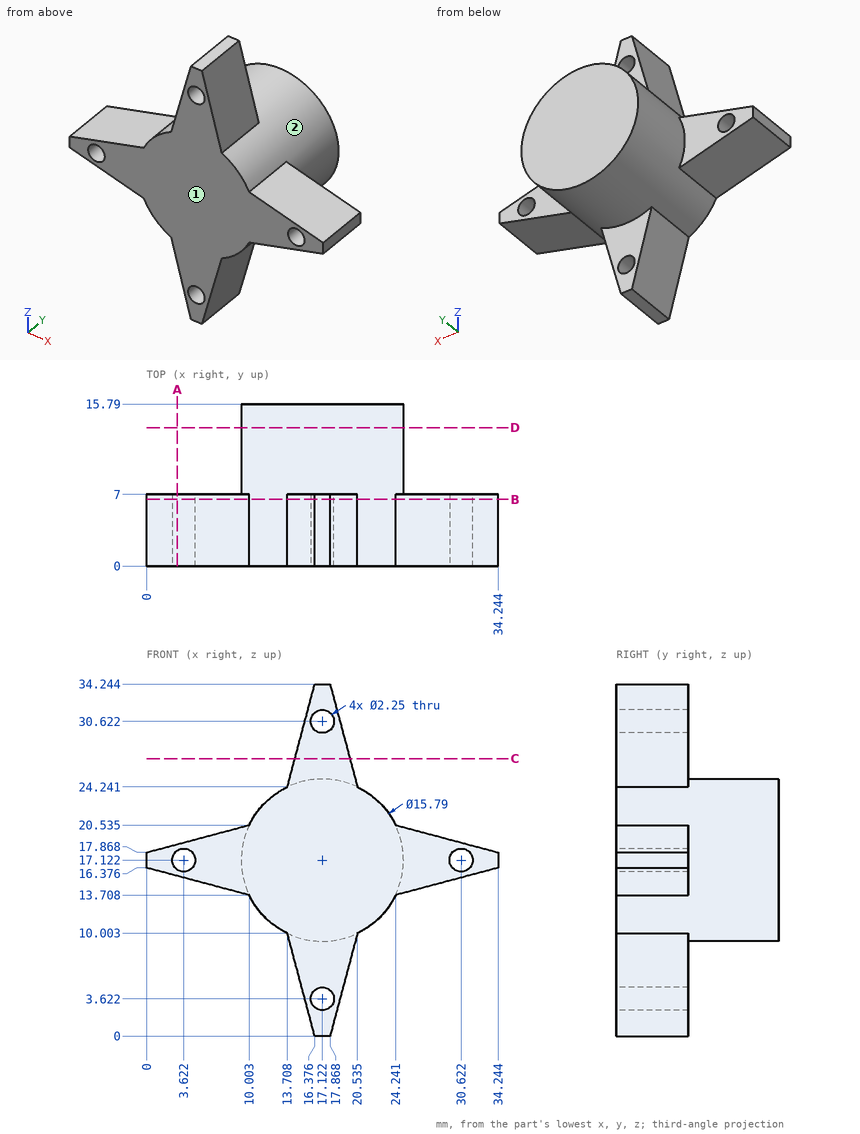
Verification items for this drawing (mm, ordinates from the low corner). A direction names the side the tool comes from. Give positions to 0.01 mm unless a question says otherwise; leave off trailing zeros. Loops run counter-clockwise (first coordinate to the right, second up) from the corner with the lowest first, then second, coordinate; pieces in that order, holes last. Notation, with made-up numbers: M 16.5,-9 L 40.5,-9 A24 ccw 40.5,27 Z; hole C 2.25,53.25 d9. An arc over 180 degrees is marked long. Return JSON: item names as keys, results as strings. Group by question number.
1. Thickness scan on L1, parallel to Y at x = 16, z = 8.5; L2, parallel to Z at x = 3, y = 2 (1 decimal); L3, parallel to X at y = 8.5, z = 12.5. Record the ranges inside material, lowest first.
2. Tool access check on the marked faces 1 and 2. Record the directions out of +Z, -Z, +X, -X, +Y, -Y that give a thin tool (end or side, any length) a straight path to the whole face; none if there is none.
3. Go/stop test with flat-tipped pins: pin 1 (5.5 mm diameter, centred on x = 18, z = 29, fed in from +Y); pin 2 (2 mm diameter, centred on x = 13.5, y = 13, fed in from +Z); pin 3 (4 mm diameter, centred on y = 11, z = 10.5, fed in from +X). Record where each tip stops, or that it passes through.
4. Cross-section at A-A on x = 3. Record the boundary of the cut face in (y, z) (1 decimal).
5. Cross-section at D-D on y = 13.5. Record the boundary of the cut face in (x, z) (1 decimal).
6. Cross-section at B-B on y = 6.5. State how many separate pieces and enclosed holes the cut face has, plus the area to 3 significant figures.
7. Cross-section at C-C on z = 27. Record the boundary of the cut face in (x, y), plus the area to 3 significant figures.
Return value:
{
 "1": {"L1": "0 to 7", "L2": "15.6 to 16.2, 18.1 to 18.7", "L3": "10.72 to 23.52"},
 "2": {"face 1": "+Z, -Z, +X, -X, -Y", "face 2": "+Y"},
 "3": {"pin 1": "y = 7", "pin 2": "z = 24.57", "pin 3": "x = 23.52"},
 "4": {"outline": "M 0,15.6 L 7,15.6 L 7,16.2 L 0,16.2 Z; M 0,18.1 L 7,18.1 L 7,18.7 L 0,18.7 Z"},
 "5": {"outline": "C 17.1,17.1 d15.8"},
 "6": {"separate pieces": "1", "enclosed holes": "4", "area": "332 mm^2"},
 "7": {"outline": "M 14.44,0 L 19.8,0 L 19.8,7 L 14.44,7 Z", "area": "37.5 mm^2"}
}
